Source: CAD feature listing. Evaluate the final solid. Frame: model axes, mm. Coordinates: 2 decimals unless noted, no trailing zeros. Loops run counter-clockwise (first coordinate to the right, second up) from the corner with the lowest first, then second, coordinate; pieces in that order, holes last. Notation, with made-up numbers: (17.5, 15.5) -> (42.5, 15.5) arc R27 cw to (42.5, 35.5) -> close; hole circle Ø7 at (86.25, 60). An arc over 180 degrees is marked (long way). Answer as CSV lines item,"result".
from build123d import *

# Parameters (mm, degrees)
CROQUIS2_R              = 112.5
SALIENTE_EXTRUIR1_DEPTH = 3
CORTAR_EXTRUIR1_REACH   = 161.127
CROQUIS3_R              = 1
CORTAR_EXTRUIR2_DEPTH   = 0.1


with BuildPart() as part:
    # Croquis2 → Saliente-Extruir1 (new body)
    with BuildSketch(Plane(origin=(0, 0, 0), x_dir=(1, 0, 0), z_dir=(0, 1, 0))):
        with Locations(Location((0, 0, 0), (0, 0, 270))):
            Circle(CROQUIS2_R)
    extrude(amount=SALIENTE_EXTRUIR1_DEPTH)

    # Croquis3 → Cortar-Extruir1 (cut, up to next)
    with BuildSketch(Plane(origin=(0, 3, 0), x_dir=(1, 0, 0), z_dir=(0, 1, 0)), mode=Mode.PRIVATE) as cortar_extruir1_sk1:
        with Locations(Location((0, 0, 0), (0, 0, 270))):
            Circle(CROQUIS3_R)
    cortar_extruir1_tool1 = extrude(cortar_extruir1_sk1.sketch, amount=-CORTAR_EXTRUIR1_REACH, mode=Mode.PRIVATE) & part.part
    add(cortar_extruir1_tool1.solids().sort_by_distance((0, 3, 0))[0], mode=Mode.SUBTRACT)

    # Croquis4 → Cortar-Extruir2 (cut)
    with BuildSketch(Plane(origin=(0, 3, 0), x_dir=(1, 0, 0), z_dir=(0, 1, 0))):
        Polygon((26.671111852, 45.340890148), (34.044889835, 52.714668131), (56.793779355, 29.96577861), (63.853779551, 37.025778806), (66.91311297, 12.472667013), (44.242667896, 17.41466715), (49.612104379, 22.784103634), align=None)
    extrude(amount=-CORTAR_EXTRUIR2_DEPTH, mode=Mode.SUBTRACT)


solid = part.part
(1) Cut plane A-A (y = 0.45). Return the cut outline in (x, z), then the cut area to 3 significant figures.
Computed values:
outline,"circle Ø225 at (0, 0); hole circle Ø2 at (0, 0)"
area,"39,800 mm^2"
(2) Material intervals for L1, parallel to X at y = 1.1, z = 0; L2, parallel to Z at x = 3.5, y = 2; L3, parallel to X at y = 2.5, z = -60, sorted ascending. Write a range as [from, to].
Computed values:
L1,"[-112.5, -1], [1, 112.5]"
L2,"[-112.45, 112.45]"
L3,"[-95.16, 95.16]"
(3) Cut plane C-C (z = 28.5). Return the cut outline in (x, y).
Computed values:
outline,"(-108.83, 0) -> (108.83, 0) -> (108.83, 3) -> (-108.83, 3) -> close"
(4) Pin query (flat end, axial travel): pin 1 Ø1.5 at (y, z) = (2, 52) entering from -X. Return the tip coordinate at first contact, or that it passes through.
Computed values:
pin 1,"x = -100.15"
(5) Cut plane B-B (x = -32.5). Return the cut outline in (y, z), then the cut area to 3 significant figures.
Computed values:
outline,"(0, -107.7) -> (3, -107.7) -> (3, 107.7) -> (0, 107.7) -> close"
area,"646 mm^2"
